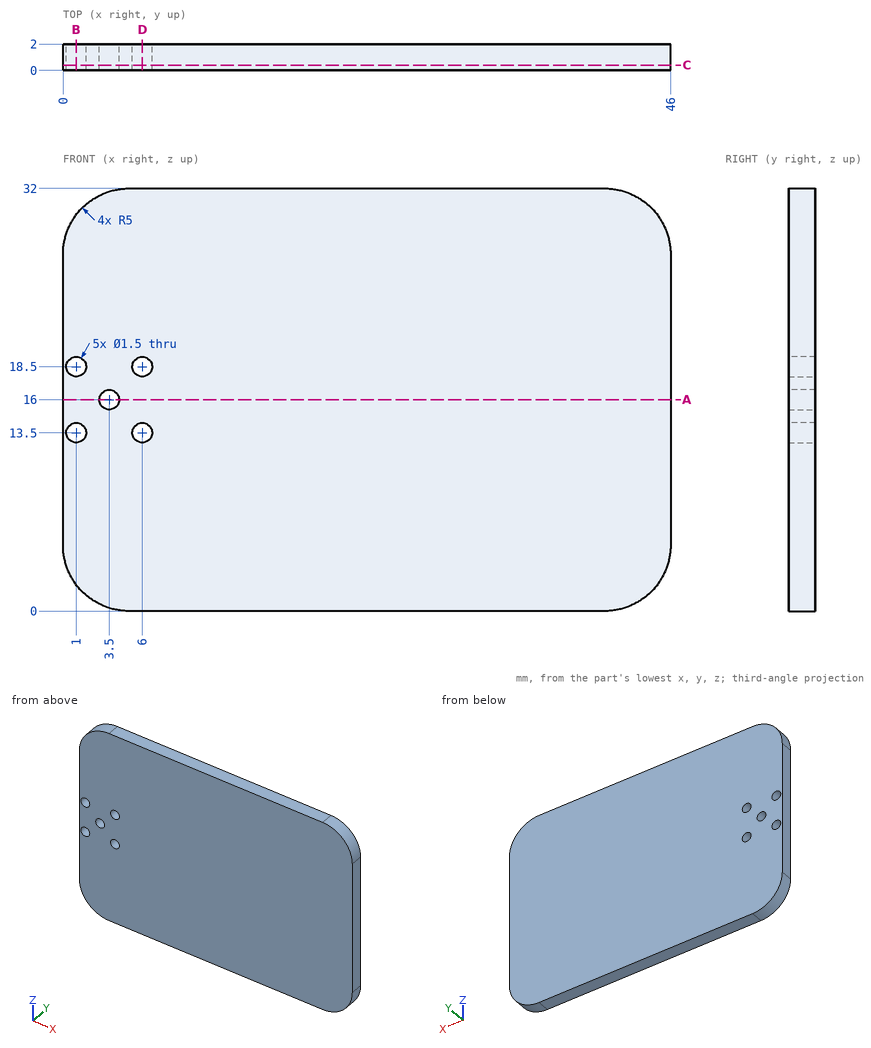
Design review of the part shown in the three views and the two pictorial views. Dimensions are in mm from the part's minimum x, y and z. Give positions to 0.01 mm unless a question says otherwise; leave off trailing zeros. Write each loop counter-clockwise with the first axis right and the second up, starting at its lowest first coordinate (ties: lowest second). Pieces come first, ordered by that corner, then holes.
(1) Wall thickness on line 1 along X through (y, z) = (0.8, 13.5); line 2 along X through (y, z) = (1.2, 18); line 3 along X through (y, z) = (1.3, 4): over which ranges is each line inside the solid? List them lowest first.
Checked values:
line 1: x = 0 to 0.25, 1.75 to 5.25, 6.75 to 46
line 2: x = 0 to 0.44, 1.56 to 5.44, 6.56 to 46
line 3: x = 0.1 to 45.9
(2) Add section A-A (z = 16). Give the boundary of the cut face in (x, y).
Checked values:
outline: (0, 0) - (2.75, 0) - (2.75, 2) - (0, 2) - close; (4.25, 0) - (46, 0) - (46, 2) - (4.25, 2) - close
(3) Add section C-C (y = 0.4). Give the boundary of the cut face in (x, z), and give its area (3 significant figures).
Checked values:
outline: (0, 5) arc R5 ccw to (5, 0) - (41, 0) arc R5 ccw to (46, 5) - (46, 27) arc R5 ccw to (41, 32) - (5, 32) arc R5 ccw to (0, 27) - close; hole circle Ø1.5 at (1, 13.5); hole circle Ø1.5 at (1, 18.5); hole circle Ø1.5 at (3.5, 16); hole circle Ø1.5 at (6, 13.5); hole circle Ø1.5 at (6, 18.5)
area: 1,440 mm2
(4) Add section B-B (x = 1). Give the boundary of the cut face in (y, z), and give its area (3 significant figures).
Checked values:
outline: (0, 2) - (2, 2) - (2, 12.75) - (0, 12.75) - close; (0, 14.25) - (2, 14.25) - (2, 17.75) - (0, 17.75) - close; (0, 19.25) - (2, 19.25) - (2, 30) - (0, 30) - close
area: 50.0 mm2
(5) Add section D-D (x = 6). Give the boundary of the cut face in (y, z), and give its area (3 significant figures).
Checked values:
outline: (0, 0) - (2, 0) - (2, 12.75) - (0, 12.75) - close; (0, 14.25) - (2, 14.25) - (2, 17.75) - (0, 17.75) - close; (0, 19.25) - (2, 19.25) - (2, 32) - (0, 32) - close
area: 58.0 mm2
